from build123d import *

# Parameters (mm, degrees)
ESQUISSE1_W             = 10
ESQUISSE1_H             = 24
BOSS_EXTRU_1_DEPTH      = 8
ESQUISSE2_W             = 51.367722688
ESQUISSE2_H             = 8
ESQUISSE2_W_2           = 58
ESQUISSE2_H_2           = 7.931606273
ENL_V_MAT_EXTRU_1_DEPTH = 4
ESQUISSE3_R             = 0.5
ESQUISSE3_R_2           = 1
ENL_V_MAT_EXTRU_2_DEPTH = 4


with BuildPart() as part:
    # Esquisse1 → Boss.-Extru.1 (new body)
    with BuildSketch(Plane.XY):
        with BuildLine():
            Line((30.577007139, 186.135890651), (30.577007139, 224.014570308))
            Line((30.577007139, 224.014570308), (-19.422992861, 224.014570308))
            Line((-19.422992861, 224.014570308), (-19.422992861, 208.014570308))
            Line((-19.422992861, 208.014570308), (15.577007139, 208.014570308))
            Line((15.577007139, 208.014570308), (15.577007139, 184.014570308))
            Line((15.577007139, 184.014570308), (-19.422992861, 184.014570308))
            Line((-19.422992861, 184.014570308), (-19.422992861, 168.014570308))
            Line((-19.422992861, 168.014570308), (15.577007139, 168.014570308))
            Line((15.577007139, 168.014570308), (15.577007139, 144.014570308))
            Line((15.577007139, 144.014570308), (-19.422992861, 144.014570308))
            Line((-19.422992861, 144.014570308), (-19.422992861, 128.014570308))
            Line((-19.422992861, 128.014570308), (15.577007139, 128.014570308))
            Line((15.577007139, 128.014570308), (15.577007139, 104.014570308))
            Line((15.577007139, 104.014570308), (-19.422992861, 104.014570308))
            Line((-19.422992861, 104.014570308), (-19.422992861, 88.014570308))
            Line((-19.422992861, 88.014570308), (15.577007139, 88.014570308))
            Line((15.577007139, 88.014570308), (15.577007139, 64.014570308))
            Line((15.577007139, 64.014570308), (-19.422992861, 64.014570308))
            Line((-19.422992861, 64.014570308), (-19.422992861, 48.014570308))
            Line((-19.422992861, 48.014570308), (15.577007139, 48.014570308))
            Line((15.577007139, 48.014570308), (15.577007139, 24.014570308))
            Line((15.577007139, 24.014570308), (-19.422992861, 24.014570308))
            Line((-19.422992861, 24.014570308), (-19.422992861, -31.985429692))
            Line((-19.422992861, -31.985429692), (30.577007139, -31.985429692))
            Line((30.577007139, -31.985429692), (38.577007139, -31.985429692))
            Line((38.577007139, -31.985429692), (38.577007139, 18.014570308))
            Line((38.577007139, 18.014570308), (32.698327483, 18.014570308))
            ThreePointArc((32.698327483, 18.014570308), (30.577007139, 18.014570308), (30.577007139, 20.135890651))
            Line((30.577007139, 20.135890651), (30.577007139, 131.893249964))
            ThreePointArc((30.577007139, 131.893249964), (30.577007139, 134.014570308), (32.698327483, 134.014570308))
            Line((32.698327483, 134.014570308), (38.577007139, 134.014570308))
            Line((38.577007139, 134.014570308), (38.577007139, 184.014570308))
            Line((38.577007139, 184.014570308), (32.698327483, 184.014570308))
            ThreePointArc((32.698327483, 184.014570308), (30.577007139, 184.014570308), (30.577007139, 186.135890651))
        make_face()
        with Locations((17.577007139, -3.985429692)):
            Rectangle(ESQUISSE1_W, ESQUISSE1_H, mode=Mode.SUBTRACT)
    extrude(amount=BOSS_EXTRU_1_DEPTH)

    # Esquisse2 → Enlèv. mat.-Extru.1 (cut)
    with BuildSketch(Plane(origin=(0, 0, 0), x_dir=(-1, 0, 0), z_dir=(0, 0, -1))):
        with BuildLine():
            Line((19.422992861, 172.014570308), (-28.510535818, 172.014570308))
            ThreePointArc((-28.510535818, 172.014570308), (-30.446580511, 172.195764547), (-30.577007139, 174.135890651))
            Line((-30.577007139, 174.135890651), (-30.577007139, 177.893249964))
            ThreePointArc((-30.577007139, 177.893249964), (-30.446580511, 179.833376068), (-28.510535818, 180.014570308))
            Line((-28.510535818, 180.014570308), (19.422992861, 180.014570308))
            Line((19.422992861, 180.014570308), (19.422992861, 172.014570308))
        make_face()
        with BuildLine():
            Line((19.422992861, 140.014570308), (-18.455686796, 140.014570308))
            ThreePointArc((-18.455686796, 140.014570308), (-20.577007139, 140.014570308), (-20.577007139, 137.893249964))
            Line((-20.577007139, 137.893249964), (-20.577007139, 134.135890651))
            ThreePointArc((-20.577007139, 134.135890651), (-20.577007139, 132.014570308), (-18.455686796, 132.014570308))
            Line((-18.455686796, 132.014570308), (19.422992861, 132.014570308))
            Line((19.422992861, 132.014570308), (19.422992861, 140.014570308))
        make_face()
        with BuildLine():
            Line((19.422992861, 100.014570308), (-18.455686796, 100.014570308))
            ThreePointArc((-18.455686796, 100.014570308), (-20.577007139, 100.014570308), (-20.577007139, 97.893249964))
            Line((-20.577007139, 97.893249964), (-20.577007139, 94.135890651))
            ThreePointArc((-20.577007139, 94.135890651), (-20.577007139, 92.014570308), (-18.455686796, 92.014570308))
            Line((-18.455686796, 92.014570308), (19.422992861, 92.014570308))
            Line((19.422992861, 92.014570308), (19.422992861, 100.014570308))
        make_face()
        with BuildLine():
            Line((19.422992861, 60.014570308), (-18.455686796, 60.014570308))
            ThreePointArc((-18.455686796, 60.014570308), (-20.577007139, 60.014570308), (-20.577007139, 57.893249964))
            Line((-20.577007139, 57.893249964), (-20.577007139, 54.135890651))
            ThreePointArc((-20.577007139, 54.135890651), (-20.577007139, 52.014570308), (-18.455686796, 52.014570308))
            Line((-18.455686796, 52.014570308), (19.422992861, 52.014570308))
            Line((19.422992861, 52.014570308), (19.422992861, 60.014570308))
        make_face()
        with BuildLine():
            Line((19.422992861, 20.014570308), (-18.455686796, 20.014570308))
            ThreePointArc((-18.455686796, 20.014570308), (-20.577007139, 20.014570308), (-20.577007139, 17.893249964))
            Line((-20.577007139, 17.893249964), (-20.577007139, 14.135890651))
            ThreePointArc((-20.577007139, 14.135890651), (-20.577007139, 12.014570308), (-18.455686796, 12.014570308))
            Line((-18.455686796, 12.014570308), (19.422992861, 12.014570308))
            Line((19.422992861, 12.014570308), (19.422992861, 20.014570308))
        make_face()
        with Locations((-6.260868483, 216.014570308)):
            Rectangle(ESQUISSE2_W, ESQUISSE2_H)
        with Locations((-9.577007139, -24.019626556)):
            Rectangle(ESQUISSE2_W_2, ESQUISSE2_H_2)
    extrude(amount=-ENL_V_MAT_EXTRU_1_DEPTH, mode=Mode.SUBTRACT)

    # Esquisse3 → Enlèv. mat.-Extru.2 (cut)
    with BuildSketch(Plane(origin=(0, 0, 4), x_dir=(-1, 0, 0), z_dir=(0, 0, -1))):
        with Locations((-15.577007139, 216.014570308)):
            Circle(ESQUISSE3_R)
        with Locations((4.922992861, -24.019626556)):
            Circle(ESQUISSE3_R_2)
        with Locations(Location((-24.077007139, -24.019626556, 0), (0, 0, 180))):
            Circle(ESQUISSE3_R_2)
    extrude(amount=-ENL_V_MAT_EXTRU_2_DEPTH, mode=Mode.SUBTRACT)


solid = part.part
Design review of the part built by this model. Coordinates are the model's own, in mm. A direction names the side the tool comes from. Coordinates: 2 decimals unless noted, no trailing zeros. Order: outer loops, then holes, each group sorted by start corner. A loop starts at its lowest first (then second) coordinate and runs counter-clockwise, first axis right, second up.
Item 1: The part is to be moulded in two halves that separate along Y. For faces 6 (the flat face through (-19.423, 216, 5)), 7 (the flat face through (6, 224.015, 4)), 8 (the flat face through (-2, 208.015, 4)), say which applies: pulls with the +Y half, pulls with the -Y half, needs draft (parallel to the pull), parting line crosses it, or undercut.
Item 2: For pin 1 Ø5 at (x, y) = (-13.5, -5) entering from -Z; pin 2 Ø2.5 at (x, y) = (12, 216) entering from -Z; pin 3 Ø1.1 at (y, z) = (135, 2.5) entering from -X, all flat-tipped, find the tip position at first contact; note any pin that passes through.
Item 3: Take a section at A-A, the plane y = 1.5. Write out the cut boundary in (x, z).
Item 4: For faces 1 (the flat face through (38.577, 159, 4)), 2 (the flat face through (6, 216, 4)), 3 (the flat face through (-19.423, 136, 5)), 4 (the flat face through (-1, 140.015, 2)), 5 (the flat face through (-2, 24.015, 4)), list the 3-axis set-ups (+Z, -Z, +X, -X, +Y, -Y) from which the entire face can be reached by the end or side of a thin tool; tool diameter is ignored.
Item 5: Take a section at D-D, the plane y = 66.5. Write out the cut boundary in (x, z).
Item 6: For line 1 (Y direction, x = -16, z = 7.75); line 2 (X direction, y = -8, z = 2.75); line 3 (Y direction, x = 17.5, z = 5.75), list the stretches that pass through material, from the lowest coordinate up.
Item 7: Take a section at B-B, the plane z = 2. Count the separate pieces of the cut face and the enclosed holes in it, then the cut area to 3 significant figures.
The answers:
1. face 6: needs draft
1. face 7: pulls with the +Y half
1. face 8: undercut
2. pin 1: stops at z = 0
2. pin 2: stops at z = 4
2. pin 3: stops at x = 20.58
3. outline: (-19.42, 0) - (12.58, 0) - (12.58, 8) - (-19.42, 8) - close; (22.58, 0) - (38.58, 0) - (38.58, 8) - (22.58, 8) - close
4. face 1: +Z, -Z, +X, +Y, -Y
4. face 2: -Z, +X, -X
4. face 3: +Z, -Z, -X, +Y, -Y
4. face 4: -Z, -X
4. face 5: +Z, -Z, -X
5. outline: (15.58, 0) - (30.58, 0) - (30.58, 8) - (15.58, 8) - close
6. line 1: y = -31.99 to 24.01, 48.01 to 64.01, 88.01 to 104.01, 128.01 to 144.01, 168.01 to 184.01, 208.01 to 224.01
6. line 2: x = -19.42 to 12.58, 22.58 to 38.58
6. line 3: y = -31.99 to -15.99, 8.01 to 224.01
7. separate pieces: 3
7. enclosed holes: 1
7. area: 6,600 mm2
